from build123d import *

# Parameters (mm, degrees)
SKETCH1_W                                 = 25.4
SKETCH1_H                                 = 50.8
SKETCH1_W_2                               = 20.32
SKETCH1_H_2                               = 45.72
VERSAFRAME_VERSAFRAME_2_X_1_X_0_1_1_DEPTH = 76.2


with BuildPart() as part:
    # Sketch1 → Versaframe VERSAFRAME 2 X 1 X 0.1 (1) (new body)
    with BuildSketch(Plane.YZ.offset(-38.1)):
        Rectangle(SKETCH1_W, SKETCH1_H)
        Rectangle(SKETCH1_W_2, SKETCH1_H_2, mode=Mode.SUBTRACT)
    extrude(amount=VERSAFRAME_VERSAFRAME_2_X_1_X_0_1_1_DEPTH)


solid = part.part
Model file for the job. Use its own axes, mm. A direction names the side the tool comes from. Round coordinates to 2 decimals unless told otherwise and drop trailing zeros. Loops run counter-clockwise (first coordinate to the right, second up) from the corner with the lowest first, then second, coordinate; pieces in that order, holes last. Notation, with made-up numbers: (-30.5, 28.25) - (2.5, 28.25) arc R7 ccw to (2.5, 41.25) - close; hole circle Ø8 at (-6, 65). An arc over 180 degrees is marked (long way). Write each question's results on one line, items separated by ' | '.
(1) 3-axis set-ups, long thin cutter, end or side, ignore diameter. For faces 4 (the flat face through (-1, 0, -25.4)), 5 (the flat face through (-1, 0, -22.86)): which of +Z, -Z, +X, -X, +Y, -Y reach the whole face in a straight line?
Answer below:
face 4: -Z, +X, -X, +Y, -Y | face 5: +X, -X
(2) Saw through at C-C, the plane x = 0. List the corners of the cut face in (y, z).
Answer below:
outline: (-12.7, -25.4) - (12.7, -25.4) - (12.7, 25.4) - (-12.7, 25.4) - close; hole (-10.16, -22.86) - (10.16, -22.86) - (10.16, 22.86) - (-10.16, 22.86) - close
(3) Saw through at A-A, the plane z = -9. List the corners of the cut face in (x, y).
Answer below:
outline: (-38.1, -12.7) - (38.1, -12.7) - (38.1, -10.16) - (-38.1, -10.16) - close; (-38.1, 10.16) - (38.1, 10.16) - (38.1, 12.7) - (-38.1, 12.7) - close
(4) Wall check: L1, parallel to Z at x = -10.5, y = -1; L2, parallel to Y at x = 35, z = 14.5. Give the ranges that are in metal, low to high.
Answer below:
L1: z = -25.4 to -22.86, 22.86 to 25.4 | L2: y = -12.7 to -10.16, 10.16 to 12.7
(5) Mould opens along Y. For faces 1 (the flat face through (-1, 12.7, 0)), 2 (the flat face through (-1, 0, 22.86)), 3 (the flat face through (-1, -12.7, 0)) say: released by +Y, released by -Y, zero draft, split by the parting line, or undercut.
Answer below:
face 1: released by +Y | face 2: undercut | face 3: released by -Y
(6) Saw through at B-B, the plane y = 6.75. List the corners of the cut face in (x, z).
Answer below:
outline: (-38.1, -25.4) - (38.1, -25.4) - (38.1, -22.86) - (-38.1, -22.86) - close; (-38.1, 22.86) - (38.1, 22.86) - (38.1, 25.4) - (-38.1, 25.4) - close
